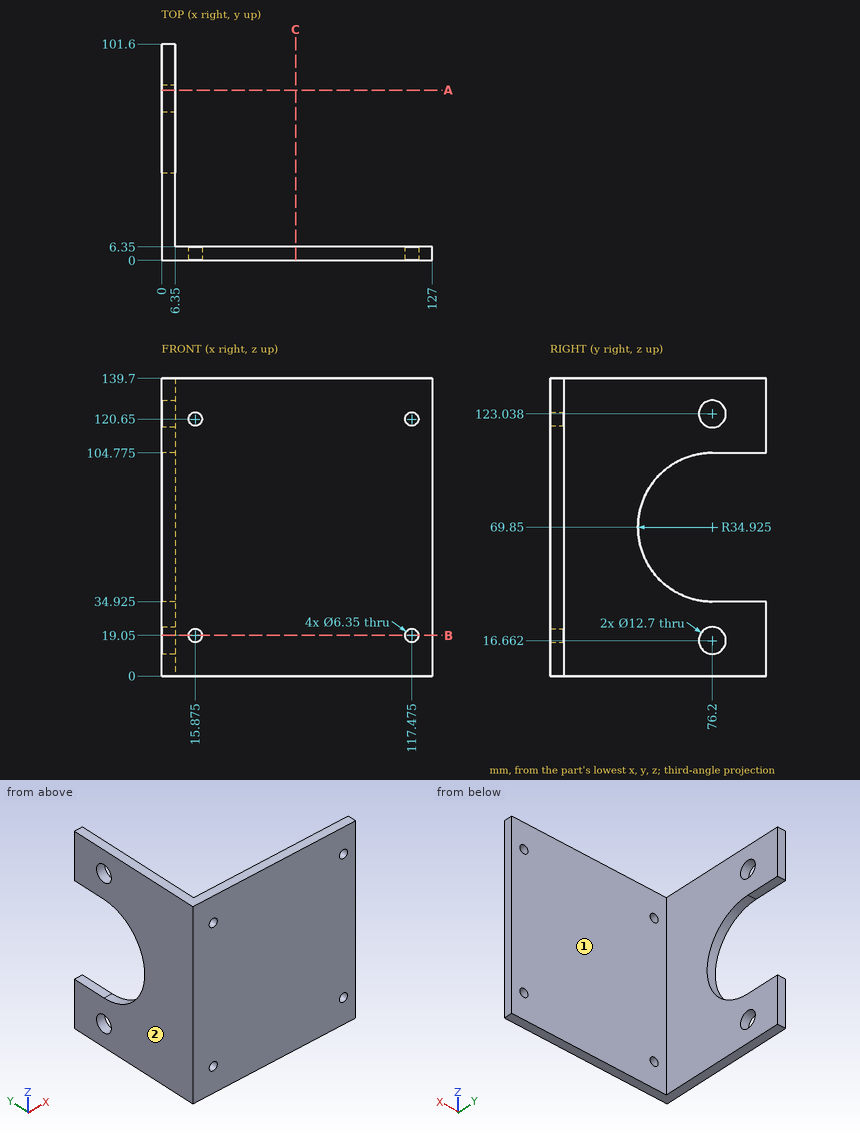
Check sheet for the drawn part. Datum: minimum x, y, z corner. Units: mm. A direction names the side the tool comes from. Round coordinates to 2 decimals unless told otherwise and drop trailing zeros. Loops run counter-clockwise (first coordinate to the right, second up) from the corner with the lowest first, then second, coordinate; pieces in that order, holes last.
Item 1: Cross-section at C-C on x = 63. Record the boundary of the cut face in (y, z).
Item 2: Gauge pin test, flat ends, axial feed: pin 1 (10 mm diameter, centred on x = 82.5, z = 86.5, fed in from +Y); pin 2 (5 mm diameter, centred on y = 75, z = 27, fed in from +X). Record the tip position at first contact, or that the pin passes through.
Item 3: Thickness scan on line 1 (X direction, y = 3.5, z = 19.05); line 2 (Y direction, x = 111.5, z = 58). Record the ranges inside material, lowest first.
Item 4: Access from +Z, -Z, +X, -X, +Y, -Y to the whole of each face (thin tool, end or side, straight path). Record for the marked faces 1 and 2.
Item 5: Cross-section at B-B on z = 19.05. Record the boundary of the cut face in (x, y), then the cut area to 3 significant figures.
Item 6: Cross-section at A-A on y = 80. Count the separate pieces of the cut face and the enclosed holes in it, then the cut area to 3 significant figures.
Answer sheet:
1. outline: (0, 0) - (6.35, 0) - (6.35, 139.7) - (0, 139.7) - close
2. pin 1: stops at y = 6.35
2. pin 2: stops at x = 6.35
3. line 1: x = 0 to 12.7, 19.05 to 114.3, 120.65 to 127
3. line 2: y = 0 to 6.35
4. face 1: +Z, -Z, +X, +Y
4. face 2: +Z, -Z, -X, +Y, -Y
5. outline: (0, 0) - (12.7, 0) - (12.7, 6.35) - (6.35, 6.35) - (6.35, 70.32) - (0, 70.32) - close; (0, 82.08) - (6.35, 82.08) - (6.35, 101.6) - (0, 101.6) - close; (19.05, 0) - (114.3, 0) - (114.3, 6.35) - (19.05, 6.35) - close; (120.65, 0) - (127, 0) - (127, 6.35) - (120.65, 6.35) - close
5. area: 1,260 mm2
6. separate pieces: 4
6. enclosed holes: 0
6. area: 314 mm2
